Geometry check sheet. Reference: the model listing, model coordinates, mm. Face numbers are marked on the shaded views. A direction names the side the tool comes from. Round coordinates to 2 decimals unless told otherwise and drop trailing zeros. Order: outer loops, then holes, each group sorted by start corner. A loop starts at its lowest first (then second) coordinate and runs counter-clockwise, first axis right, second up.
(1) Sectioned sample at A-A (z = -25). Record the boundary of the cut face in (x, y).
(2) Release check for a two-part mould opening along Z. For the marked faces 1, 2 and 3 record: +Z half, -Z half, draft (parallel to the pull), parting line (faces both ways), or undercut.
(3) Sectioned sample at D-D (z = 43.5). Record the boundary of the cut face in (x, y).
(4) Set-up check for the marked faces 4 and 5: record each of +Z, -Z, +X, -X, +Y, -Y from which the full face is reachable in a straight line by a thin tool's end or side.
(5) Sectioned sample at B-B (y = -24.5). Record the boundary of the cut face in (x, z), plus the area to 3 significant figures.
(6) Sectioned sample at C-C (x = -84.5). Record the boundary of the cut face in (y, z), plus the area to 3 significant figures.
(7) Go/stop test with flat-tipped pins: pin 1 (1.2 mm diameter, centred on x = -38.5, y = 14, fed in from +Z); pin 2 (24.5 mm diameter, centred on x = -76, y = 16.5, fed in from -Z); pin 3 (1.5 mm diameter, centred on y = 26, z = 26.5, fed in from -X). Record where each tip stops, or that it passes through.
(8) Material ranges on line 1 along Z through (x, y) = (-123, 37); line 2 along X through (y, z) = (11, -1.5); line 3 along Z through (x, y) = (-120, -14.5), recorded low to high.
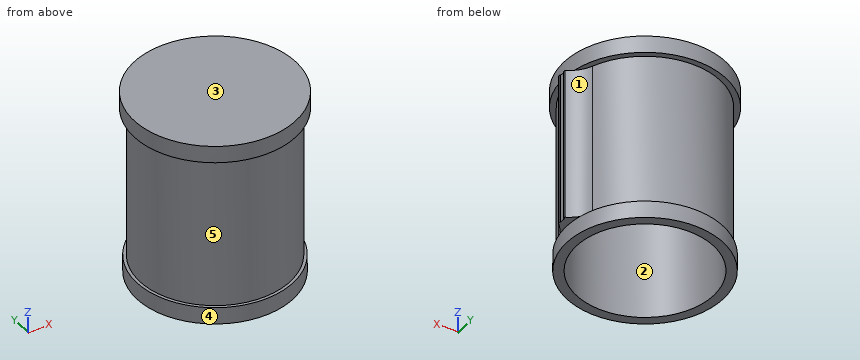
from build123d import *

# Parameters (mm, degrees)
CROQUIS1_R              = 44.422335488
SALIENTE_EXTRUIR1_DEPTH = 50
CROQUIS2_R              = 46.199565805
SALIENTE_EXTRUIR2_DEPTH = 10
CROQUIS3_R              = 47.848668402
SALIENTE_EXTRUIR3_DEPTH = 10
CROQUIS5_R              = 40.518185266
CORTAR_EXTRUIR4_DEPTH   = 105
CROQUIS8_W              = 90
CROQUIS8_H              = 6.022343016
SALIENTE_EXTRUIR4_DEPTH = 45.5
CROQUIS9_W              = 59.465557631
CROQUIS9_H              = 90
CORTAR_EXTRUIR5_DEPTH   = 45
CROQUIS10_W             = 22.822208634
CROQUIS10_H             = 90
CORTAR_EXTRUIR6_DEPTH   = 45
CROQUIS11_W             = 90
CROQUIS11_H             = 3.447121101
CORTAR_EXTRUIR7_DEPTH   = 0.5
REDONDEO1_R             = 20
REDONDEO2_R             = 40


with BuildPart() as part:
    # Croquis1 → Saliente-Extruir1 (new, symmetric)
    with BuildSketch(Plane(origin=(0, 9.520016683, 0), x_dir=(1, 0, 0), z_dir=(0, 0, 1))):
        with Locations(Location((-87.884188046, 0, 0), (0, 0, 180))):
            Circle(CROQUIS1_R)
    extrude(amount=SALIENTE_EXTRUIR1_DEPTH, both=True)

    # Croquis2 → Saliente-Extruir2 (add)
    with BuildSketch(Plane(origin=(0, 9.520016683, -50), x_dir=(-1, 0, 0), z_dir=(0, 0, -1))):
        with Locations((87.884188046, 0)):
            Circle(CROQUIS2_R)
    extrude(amount=SALIENTE_EXTRUIR2_DEPTH)

    # Croquis3 → Saliente-Extruir3 (add)
    with BuildSketch(Plane(origin=(0, 9.520016683, 50), x_dir=(1, 0, 0), z_dir=(0, 0, 1))):
        with Locations((-87.884188046, 0)):
            Circle(CROQUIS3_R)
    extrude(amount=-SALIENTE_EXTRUIR3_DEPTH)

    # Croquis5 → Cortar-Extruir4 (cut)
    with BuildSketch(Plane(origin=(0, 9.520016683, -60), x_dir=(-1, 0, 0), z_dir=(0, 0, -1))):
        with Locations((87.884188046, 0)):
            Circle(CROQUIS5_R)
    extrude(amount=-CORTAR_EXTRUIR4_DEPTH, mode=Mode.SUBTRACT)

    # Croquis8 → Saliente-Extruir4 (add, symmetric)
    with BuildSketch(Plane(origin=(0, 0, 0), x_dir=(0, 0, -1), z_dir=(1, 0, 0))):
        with Locations((5, 12.531188191)):
            Rectangle(CROQUIS8_W, CROQUIS8_H)
    extrude(amount=SALIENTE_EXTRUIR4_DEPTH, both=True)

    # Croquis9 → Cortar-Extruir5 (cut)
    with BuildSketch(Plane(origin=(0, 15.542359699, 0), x_dir=(1, 0, 0), z_dir=(0, 1, 0))):
        with Locations((15.767221184, 5)):
            Rectangle(CROQUIS9_W, CROQUIS9_H)
    extrude(amount=-CORTAR_EXTRUIR5_DEPTH, mode=Mode.SUBTRACT)

    # Croquis10 → Cortar-Extruir6 (cut)
    with BuildSketch(Plane(origin=(0, 15.542359699, 0), x_dir=(1, 0, 0), z_dir=(0, 1, 0))):
        with Locations((-25.376661948, 5)):
            Rectangle(CROQUIS10_W, CROQUIS10_H)
    extrude(amount=-CORTAR_EXTRUIR6_DEPTH, mode=Mode.SUBTRACT)

    # Croquis11 → Cortar-Extruir7 (cut)
    with BuildSketch(Plane(origin=(-36.787766265, 0, 0), x_dir=(0, 0, -1), z_dir=(1, 0, 0))):
        with Locations((5, 12.607575702)):
            Rectangle(CROQUIS11_W, CROQUIS11_H)
    extrude(amount=-CORTAR_EXTRUIR7_DEPTH, mode=Mode.SUBTRACT)

    # Redondeo1
    # the kernel refuses this fillet: 20 mm, written as the material it adds along each edge
    with BuildSketch(Plane(origin=(-43.871970711, 15.542359699, -50), x_dir=(-0.25635201555955867, 0.966583490505891, 0), z_dir=(0, 0, 1))) as redondeo1_piece_1:
        with BuildLine():
            CenterArc((13.381955248, -19.848268644), REDONDEO1_R, 97.062122585, 42.393283836)
            Line((-1.816050088, -6.847475061), (-2.120010195, -6.587459189))
            ThreePointArc((-2.120010195, -6.587459189), (-1.29465844, -3.321196724), (-0.386633396, 0.102540806))
            Line((-0.386633396, 0.102540806), (0.049178173, 0.396965373))
            ThreePointArc((0.049178173, 0.396965373), (5.46152329, 0.06298694), (10.873868406, 0.396965373))
            Line((10.873868406, 0.396965373), (10.92304658, 0))
        make_face()
    extrude(amount=90)

    # Redondeo2
    # the kernel refuses this fillet: 40 mm, written as the material it adds along each edge
    with BuildSketch(Plane(origin=(-43.461852558, 9.520016683, -50), x_dir=(1, 0, 0), z_dir=(0, 0, 1))) as redondeo2_piece_1:
        with BuildLine():
            CenterArc((35.211176648, -28.029171841), REDONDEO2_R, 135.514455154, 25.094644296)
            Line((-2.519839285, -14.748718663), (-3.274459604, -14.483109599))
            ThreePointArc((-3.274459604, -14.483109599), (-1.423064565, -7.346485792), (-0.8, 0))
            Line((-0.8, 0), (0, 0.8))
            ThreePointArc((0, 0.8), (3.337043147, 0.8), (6.103344486, 0.560583437))
            Line((6.103344486, 0.560583437), (6.674086293, 0))
        make_face()
    extrude(amount=90)


solid = part.part
Answer below:
1. outline: (-46.67, 26.1) arc R44.42 ccw (long way) to (-45.98, -5.23) arc R40 cw to (-36.79, 9.52) - (-36.79, 10.88) - (-37.29, 10.88) - (-37.29, 14.33) - (-36.79, 14.33) - (-36.79, 15.54) arc R20 cw to start; hole circle Ø81.04 at (-87.88, 9.52)
2. face 1: undercut
2. face 2: draft
2. face 3: +Z half
3. outline: circle Ø95.7 at (-87.88, 9.52); hole circle Ø81.04 at (-87.88, 9.52)
4. face 4: -Z
4. face 5: none
5. outline: (-121.53, 40) - (-116.45, 40) - (-116.45, -50) - (-119.14, -50) - (-119.14, -60) - (-109.89, -60) - (-109.89, 45) - (-65.88, 45) - (-65.88, -60) - (-56.63, -60) - (-56.63, -50) - (-59.32, -50) - (-59.32, 40) - (-54.24, 40) - (-54.24, 50) - (-121.53, 50) - close
5. area: 1,820 mm2
6. outline: (-38.21, 40) - (-34.77, 40) - (-34.77, -50) - (-36.56, -50) - (-36.56, -60) - (-30.86, -60) - (-30.86, 45) - (49.9, 45) - (49.9, -60) - (55.6, -60) - (55.6, -50) - (53.81, -50) - (53.81, 40) - (57.25, 40) - (57.25, 50) - (-38.21, 50) - close
6. area: 1,370 mm2
7. pin 1: stops at z = 40
7. pin 2: stops at z = 45
7. pin 3: stops at x = -129.43
8. line 1: z = -60 to -50, 40 to 50
8. line 2: x = -132.28 to -128.38, -47.39 to -37.29
8. line 3: z = 45 to 50
